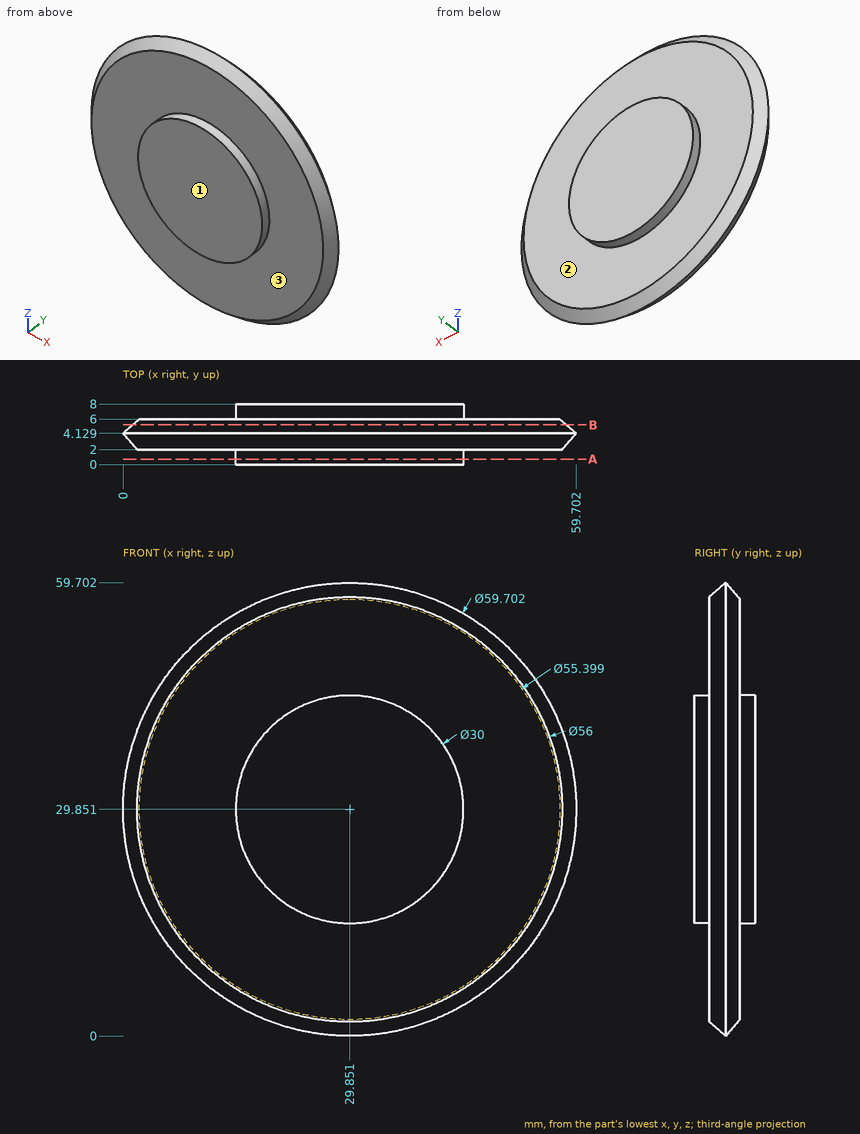
Could you check a few things on this drawing? It's one solid part, dimensions in mm from its lowest x, y, z. A direction names the side the tool comes from. Give positions to 0.01 mm unless a question says otherwise; leave off trailing zeros. Order: outer loops, then holes, each group sorted by start corner. A loop starts at its lowest first (then second) coordinate and runs counter-clockwise, first axis right, second up. Notation, with made-up numbers: (57.5, 14.5) -> (75.5, 14.5) arc R18 cw to (75.5, 28.5) -> close; hole circle Ø4 at (77.25, -6). An arc over 180 degrees is marked (long way). Answer in a Markdown table with one row per item. Add a question column.
Item 1: Imagine slicing it at A-A (y = 0.75). List the corners of the cut face in (x, z) for me, and give its area (3 significant figures).
Item 2: For the marked faces 1, 2 and 3, which set-ups out of +Z, -Z, +X, -X, +Y, -Y let a thin tool reach every point of the face, with its end or its side?
Item 3: Imagine slicing it at B-B (y = 5.25). List the corners of the cut face in (x, z) for me (1 decimal).
Item 4: Please list where these lines run through material, in increasing order: probe 1 along Y at (x, z) = (13, 48.5); probe 2 along X at (y, z) = (5, 54) (1 decimal); probe 3 along X at (y, z) = (2.25, 41.5).
Item 5: I'm going to push flat-ended pins straight in: P1, Ø1.5, axis at y = 5.5, z = 9, coming from the +X side (1 decimal); P2, Ø4, axis at x = 12.5, z = 44.5, coming from the +Y side. Where does each tip first touch, or does it pass through?
Result:
| question | item | result |
|---|---|---|
| 1 | outline | circle Ø30 at (29.85, 29.85) |
| 1 | area | 707 mm2 |
| 2 | face 1 | +Z, -Z, +X, -X, -Y |
| 2 | face 2 | +Y |
| 2 | face 3 | -Y |
| 3 | outline | circle Ø57.1 at (29.9, 29.9) |
| 4 | probe 1 | 2 to 6 |
| 4 | probe 2 | 14.1 to 45.6 |
| 4 | probe 3 | 4.15 to 55.55 |
| 5 | P1 | x = 50.4 |
| 5 | P2 | y = 6 |
